Autodesk Inventor part; units mm, degrees
ref_plane "작업 평면1" through (-13, 15, 0) normal (0, 1, 0) x (1, 0, 0)
ref_plane "작업 평면2" through (0, -5, 10) normal (1, 0, 0) x (0, 0, -1)
ref_plane "YZ Plane" through (0, 0, 0) normal (1, 0, 0) x (0, 1, 0)
sketch "스케치1" plane through (0, 0, 0) normal (0, 0, 1) x (1, 0, 0)
  line L0 (-13, -5) -> (13, -5)
  line L1 (13, -5) -> (13, 5)
  line L2 (13, 5) -> (-13, 5)
  line L3 (-13, 5) -> (-13, -5)
  line L4 (-13, -5) -> (13, 5) construction
  line L5 (13, -5) -> (-13, 5) construction
  circle A0 centre (0, 0) radius 2.5
  dimension "d0" = 26
  dimension "d1" = 10
  dimension "d2" = 5
extrude "돌출1" add sketch "스케치1" along normal blind 10
sketch "스케치2" plane through (-13, 5, 0) normal (0, 1, 0) x (1, 0, 0)
  line L0 (26, 0) -> (0, 0)
  line L1 (26, -10) -> (0, -10)
  line L2 (0, 0) -> (5, 0)
  line L3 (5, 0) -> (5, -10)
  line L4 (5, -10) -> (0, -10)
  line L5 (0, -10) -> (0, 0)
  line L6 (13, 0) -> (13, -10)
  line L7 (26, 0) -> (21, 0)
  line L8 (21, 0) -> (21, -10)
  line L9 (21, -10) -> (26, -10)
  line L10 (26, -10) -> (26, 0)
  point P0 (0, -10)
  point P1 (21, 0)
  dimension "d5" = 5
  dimension "d6" = 8
extrude "돌출2" add sketch "스케치2" along normal blind 10 contours L10 L1 L8 L0 | L3 L1 L5 L0
sketch "스케치3" plane through (-13, 5, 0) normal (-1, 0, 0) x (0, 0, 1)
  circle A0 centre (5, 5) radius 2.5
  line L0 (0, 10) -> (10, 10)
  line L1 (10, -10) -> (10, 10)
  point P0 (0, -5)
  point P1 (10, 0)
  point P2 (10, 5)
  point P3 (5, 10)
  point P4 (5, 10)
  dimension "d9" = 5
extrude "돌출3" cut sketch "스케치3" against normal through all
ref_plane "작업 평면1" through (-13, 15, 0) normal (0, 1, 0) x (1, 0, 0)
mirror "미러1" about plane through (-10.5, 15, 5) normal (0, 1, 0) of "돌출3", "돌출2"
sketch "스케치4" plane through (0, 0, 0) normal (0, 0, -1) x (-1, 0, 0)
  line L0 (-13, 5) -> (-13, 25)
  line L1 (13, -5) -> (-13, -5)
  line L2 (-13, 25) -> (13, 25)
  line L3 (13, 25) -> (13, -5)
  line L4 (13, -5) -> (-13, -5)
  line L5 (-13, -5) -> (-13, 25)
  point P0 (0, 0)
  point P1 (13, 25)
extrude "돌출4" add sketch "스케치4" along normal blind 5
ref_plane "작업 평면2" through (0, -5, 10) normal (1, 0, 0) x (0, 0, -1)
sketch "스케치5" plane through (0, -5, 10) normal (1, 0, 0) x (0, 0, -1)
  line L0 (10, 10) -> (10, 30)
  line L1 (10, 30) -> (15, 30)
  line L2 (15, 30) -> (15, 35)
  line L3 (15, 35) -> (10, 35)
  line L4 (10, 35) -> (10, 30)
  circle A0 centre (12.5, 32.5) radius 1.5
  point P0 (10, 5)
  point P1 (10, 32.5)
  point P2 (12.5, 35)
  dimension "d16" = 5
  dimension "d19" = 3
extrude "돌출5" add sketch "스케치5" along normal mid plane 15
extrude "돌출6" cut sketch "스케치5" along normal mid plane 5
fillet "모깎기2" radius 2.5 4 edges at (-5, 30, -5) (-5, 30, 0) (5, 30, -5) (5, 30, 0)
sketch "스케치6" plane through (0, 0, 10) normal (0, 0, 1) x (1, 0, 0)
  line L0 (-13, -5) -> (13, -5)
  line L1 (13, 25) -> (13, -5)
  line L2 (-13, -5) -> (13, -5)
  line L3 (13, -5) -> (13, 5)
  line L4 (13, 5) -> (-13, 5)
  line L5 (-13, 5) -> (-13, -5)
  point P0 (0, 0)
  point P1 (8, 5)
extrude "돌출7" cut sketch "스케치6" against normal through all
sketch "스케치7" plane through (-8, 5, 0) normal (0, -1, 0) x (1, 0, 0)
  circle A0 centre (8, -2.5) radius 1.5
  line L0 (16, 0) -> (0, 0)
  line L1 (21, -5) -> (-5, -5)
  point P0 (8, 0)
  point P1 (8, 0)
  dimension "d25" = 3
  dimension "d26" = 5
  dimension "d27" = 2.5
extrude "돌출8" cut sketch "스케치7" against normal through all
equation "\"d27\" = 0.5 * d26"
properties part number "SteeringFrameFront"
Design review of the part built by this model. Coordinates are the model's own, in mm. A direction names the side the tool comes from. Coordinates: 2 decimals unless noted, no trailing zeros. Loops run counter-clockwise (first coordinate to the right, second up) from the corner with the lowest first, then second, coordinate; pieces in that order, holes last. Notation, with made-up numbers: (-5.5, 9.25) -> (42.5, 9.25) arc R23 ccw to (42.5, 30.25) -> close; hole circle Ø2 at (-1, 46). An arc over 180 degrees is marked (long way). Answer as a JSON object with one key per item and string values.
Q1. Take a section at D-D on x = 0. Give the boundary of the cut face in (y, z), plus the area to 3 significant figures.
Answer block:
{"outline": "(5, -5) -> (25, -5) -> (25, -4) -> (5, -4) -> close; (5, -1) -> (25, -1) -> (25, 0) -> (5, 0) -> close", "area": "40.0 mm^2"}
Q2. The part is to be moulded in two halves that separate along X. For faces 4 (the flat face through (10, 15, 10)), 5 (the flat face through (-2.5, 26, -4)), 6 (the flat face through (13, 15, 3)), 7 (the flat face through (1, 25, -1)), say which applies: +X half, -X half, draft (parallel to the pull), parting line (faces both ways), or undercut.
Answer block:
{"face 4": "draft", "face 5": "undercut", "face 6": "+X half", "face 7": "undercut"}
Q3. Tool access review of faces 1 (the flat face through (8, 15, 5)), 2 (the flat face through (2.5, 26, -4)), 3 (the flat face through (-7.5, 26, -4)): name each direction out of +Z, -Z, +X, -X, +Y, -Y from which nothing blocks a thin tool from reaching the whole face with its end or side.
Answer block:
{"face 1": "+Z, +Y, -Y", "face 2": "+Z, -Z, +Y", "face 3": "+Z, -Z, -X, +Y"}
Q4. Clearance check with flat-ended pins moving along their axes: pin 1 Ø1.6 at (x, z) = (10, 3) entering from +Y; pin 2 Ø5 at (x, z) = (0, -2.5) entering from -Y; pin 3 Ø1 at (x, y) = (-0.5, 9.5) entering from +Z; pin 4 Ø2.5 at (y, z) = (28.5, -2) entering from +X. State where each tip first meets the part, or that it passes through.
Answer block:
{"pin 1": "stops at y = 25", "pin 2": "stops at y = 5", "pin 3": "stops at z = 0", "pin 4": "stops at x = 7.5"}
Q5. Take a section at C-C on y = 16.75. Give the boundary of the cut face in (x, z).
Answer block:
{"outline": "(-13, -5) -> (13, -5) -> (13, 10) -> (8, 10) -> (8, 0) -> (-8, 0) -> (-8, 10) -> (-13, 10) -> close; hole circle Ø3 at (0, -2.5)"}
Q6. Take a section at A-A on y = 10. Give the boundary of the cut face in (x, z).
Answer block:
{"outline": "(-13, -5) -> (13, -5) -> (13, 2.5) -> (8, 2.5) -> (8, 0) -> (-8, 0) -> (-8, 2.5) -> (-13, 2.5) -> close; (-13, 7.5) -> (-8, 7.5) -> (-8, 10) -> (-13, 10) -> close; (8, 7.5) -> (13, 7.5) -> (13, 10) -> (8, 10) -> close; hole circle Ø3 at (0, -2.5)"}
Q7. To check wall thickness, follow L1, parallel to Y at x = -11.3, z = 5; L2, parallel to Z at x = -11.55, y = 20; L3, parallel to X at y = 24.25, z = 2.5. State the ranges of each line that lie inside material, in increasing order.
Answer block:
{"L1": "y = 5 to 7.5, 12.5 to 17.5, 22.5 to 25", "L2": "z = -5 to 2.5, 7.5 to 10", "L3": "x = -13 to -8, 8 to 13"}
Q8. Take a section at B-B on z = 1.75. Give the boundary of the cut face in (x, y).
Answer block:
{"outline": "(-13, 5) -> (-8, 5) -> (-8, 25) -> (-13, 25) -> close; (8, 5) -> (13, 5) -> (13, 25) -> (8, 25) -> close"}
